Check sheet for the modelled part. Datum: model origin and axes. Units: mm. Face numbers are marked on the shaded views. A direction names the side the tool comes from. Give positions to 0.01 mm unless a question says otherwise; leave off trailing zeros. Order: outer loops, then holes, each group sorted by start corner. A loop starts at its lowest first (then second) coordinate and runs counter-clockwise, first axis right, second up.
from build123d import *

# Parameters (mm, degrees)
SKETCH1_R           = 2.38
BOSS_EXTRUDE1_DEPTH = 32.2
BOSS_EXTRUDE2_START = 0.5
SKETCH1_3_W         = 2.5
SKETCH1_3_H         = 16
BOSS_EXTRUDE2_DEPTH = 6
CUT_EXTRUDE1_START  = 32.2
SKETCH1_4_R         = 1.25
CUT_EXTRUDE1_DEPTH  = 2
BOSS_EXTRUDE3_START = 32.2
SKETCH1_5_R         = 11
SKETCH1_5_R_2       = 2.38
BOSS_EXTRUDE3_DEPTH = 2


with BuildPart() as part:
    # Sketch1 → Boss-Extrude1 (new body)
    with BuildSketch(Plane.XY):
        with BuildLine():
            Line((11.5, 14.1), (-11.5, 14.1))
            ThreePointArc((-11.5, 14.1), (-13.338477631, 13.338477631), (-14.1, 11.5))
            Line((-14.1, 11.5), (-14.1, -11.5))
            ThreePointArc((-14.1, -11.5), (-13.338477631, -13.338477631), (-11.5, -14.1))
            Line((-11.5, -14.1), (11.5, -14.1))
            ThreePointArc((11.5, -14.1), (13.338477631, -13.338477631), (14.1, -11.5))
            Line((14.1, -11.5), (14.1, 11.5))
            ThreePointArc((14.1, 11.5), (13.338477631, 13.338477631), (11.5, 14.1))
        make_face()
        Circle(SKETCH1_R, mode=Mode.SUBTRACT)
    extrude(amount=BOSS_EXTRUDE1_DEPTH)

    # Sketch1<3> → Boss-Extrude2 (add)
    with BuildSketch(Plane.XY.offset(BOSS_EXTRUDE2_START)):
        with Locations((15.35, 0)):
            Rectangle(SKETCH1_3_W, SKETCH1_3_H)
    extrude(amount=BOSS_EXTRUDE2_DEPTH)

    # Sketch1<4> → Cut-Extrude1 (cut)
    with BuildSketch(Plane.XY.offset(CUT_EXTRUDE1_START)):
        with Locations((-11.5, 11.5)):
            Circle(SKETCH1_4_R)
        with Locations((11.5, 11.5)):
            Circle(SKETCH1_4_R)
        with Locations((11.5, -11.5)):
            Circle(SKETCH1_4_R)
        with Locations((-11.5, -11.5)):
            Circle(SKETCH1_4_R)
    extrude(amount=-CUT_EXTRUDE1_DEPTH, mode=Mode.SUBTRACT)

    # Sketch1<5> → Boss-Extrude3 (add)
    with BuildSketch(Plane.XY.offset(BOSS_EXTRUDE3_START)):
        Circle(SKETCH1_5_R)
        Circle(SKETCH1_5_R_2, mode=Mode.SUBTRACT)
    extrude(amount=BOSS_EXTRUDE3_DEPTH)


solid = part.part
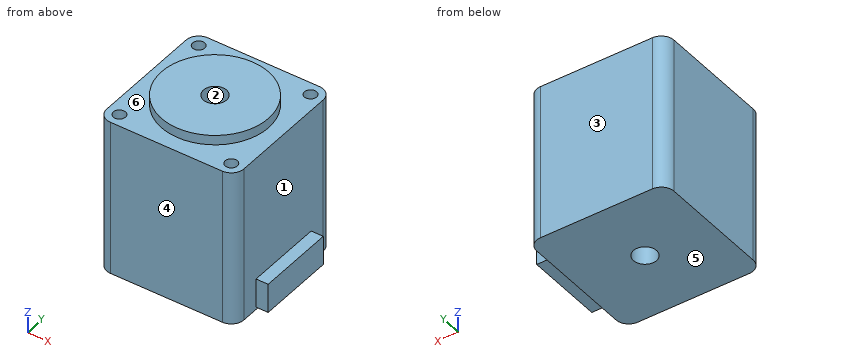
1) Section check C-C, the plane y = -9.25. Record the cut outline in (x, z), then the cut area to 3 significant figures.
Recorded:
outline: (-14.1, 0) - (14.1, 0) - (14.1, 32.2) - (5.95, 32.2) - (5.95, 34.2) - (-5.95, 34.2) - (-5.95, 32.2) - (-14.1, 32.2) - close
area: 932 mm2
2) Depth check by flat-ended pin: pin 1 Ø1.2 at (x, y) = (11, 11) entering from +Z; pin 2 Ø12 at (y, z) = (11, 21) entering from +X; pin 3 Ø2 at (x, y) = (16, -2.5) entering from +Z. Enter the tip coordinate at first touch or a pass-through.
Recorded:
pin 1: stops at z = 32.2
pin 2: stops at x = 14.1
pin 3: stops at z = 6.5
3) Material ranges on L1, parallel to Y at x = 11.5, z = 30.7; L2, parallel to Y at x = 11, z = 31; L3, parallel to Z at x = 14.5, y = 1.75, recorded low to high.
Recorded:
L1: y = -14.1 to -12.75, -10.25 to 10.25, 12.75 to 14.1
L2: y = -14.1 to -12.65, -10.35 to 10.35, 12.65 to 14.1
L3: z = 0.5 to 6.5
4) Section check B-B, the plane x = 0. Record the cut outline in (y, z).
Recorded:
outline: (-14.1, 0) - (-2.38, 0) - (-2.38, 34.2) - (-11, 34.2) - (-11, 32.2) - (-14.1, 32.2) - close; (2.38, 0) - (14.1, 0) - (14.1, 32.2) - (11, 32.2) - (11, 34.2) - (2.38, 34.2) - close
5) Set-up check for the marked faces 5 and 6: record each of +Z, -Z, +X, -X, +Y, -Y from which the full face is reachable in a straight line by a thin tool's end or side.
Recorded:
face 5: -Z, +X, -X, +Y, -Y
face 6: +Z
6) Section check A-A, the plane z = 7. Record the cut outline in (x, y).
Recorded:
outline: (-14.1, -11.5) arc R2.6 ccw to (-11.5, -14.1) - (11.5, -14.1) arc R2.6 ccw to (14.1, -11.5) - (14.1, 11.5) arc R2.6 ccw to (11.5, 14.1) - (-11.5, 14.1) arc R2.6 ccw to (-14.1, 11.5) - close; hole circle Ø4.76 at (0, 0)
7) Draft check along Y on the marked faces 1, 2, 3 and 4. Enter one of: +Y half, -Y half, draft (parallel to the pull), parting line (faces both ways), or undercut.
Recorded:
face 1: draft
face 2: undercut
face 3: +Y half
face 4: -Y half
8) Section check D-D, the plane x = 4.5. Record the cut outline in (y, z).
Recorded:
outline: (-14.1, 0) - (14.1, 0) - (14.1, 32.2) - (10.04, 32.2) - (10.04, 34.2) - (-10.04, 34.2) - (-10.04, 32.2) - (-14.1, 32.2) - close
